Read the model definition and answer for the solid it produces. Units are mm, in the model's axes. Face numbers are marked on the shaded views. Give positions to 0.01 mm unless a question says otherwise; leave off trailing zeros. Order: outer loops, then holes, each group sorted by start corner. A loop starts at its lowest first (then second) coordinate and runs counter-clockwise, first axis right, second up. Notation, with made-up numbers: M 19.25,-17 L 44.25,-17 A20 ccw 44.25,21 Z; hole C 42,21 d7. An arc over 180 degrees is marked long. Write item = value, one per line. Start each with the question number.
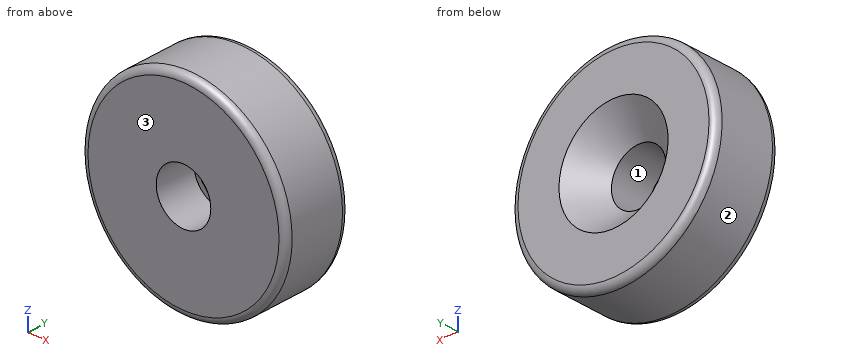
from build123d import *

# Parameters (mm, degrees)
SKETCH1_R           = 7.5
SKETCH1_R_2         = 2
BOSS_EXTRUDE1_DEPTH = 2.5
FILLET1_R           = 0.5
CHAMFER1_SIZE       = 2


with BuildPart() as part:
    # Sketch1 → Boss-Extrude1 (new body, symmetric)
    with BuildSketch(Plane(origin=(0, 0, 0), x_dir=(1, 0, 0), z_dir=(0, 1, 0))):
        Circle(SKETCH1_R)
        Circle(SKETCH1_R_2, mode=Mode.SUBTRACT)
    extrude(amount=BOSS_EXTRUDE1_DEPTH, both=True)

    # Fillet1
    fillet1_edges = [part.edges().sort_by_distance(p)[0] for p in [
        (-7.5, -2.5, 0),
        (-7.5, 2.5, 0),
    ]]
    fillet(fillet1_edges, radius=FILLET1_R)

    # Chamfer1
    chamfer1_edges = [part.edges().sort_by_distance(p)[0] for p in [
        (-2, 2.5, 0),
    ]]
    chamfer(chamfer1_edges, length=CHAMFER1_SIZE)


solid = part.part
1) Find section B-B on x = 0. Determine the outline of the cut face in (y, z), plus the area to 3 significant figures.
2) For a pull along Z with two mould halves and no side action, classify the marked faces 1, 2 and 3 as pulls with the +Z half, pulls with the -Z half, needs draft (parallel to the pull), parting line crosses it, or undercut.
3) Find the intervals of material crossed by probe 1 along X at (y, z) = (-1.05, 0); probe 2 along X at (y, z) = (1.35, 0.25), in increasing order. Write a range as [from, to].
4) Find section C-C on y = -0.45. Determine the outline of the cut face in (x, z), plus the area to 3 significant figures.
5) Find section D-D on y = 1.75. Determine the outline of the cut face in (x, z), plus the area to 3 significant figures.
6) Each of these flat-tipped pins is pushed along its axis until it touches: P1, Ø3, axis at y = -1, z = -6, coming from the +X side; P2, Ø2, axis at x = -4.5, y = 1.5, coming from the +Z side. Where does it stop, or does it pass through?
7) Find section A-A on z = 0. Determine the outline of the cut face in (x, y), plus the area to 3 significant figures.
Numbers:
q1.outline = M -2.5,-7 A0.5 ccw -2,-7.5 L 2,-7.5 A0.5 ccw 2.5,-7 L 2.5,-4 L 0.5,-2 L -2.5,-2 Z; M -2.5,2 L 0.5,2 L 2.5,4 L 2.5,7 A0.5 ccw 2,7.5 L -2,7.5 A0.5 ccw -2.5,7 Z
q1.area = 50.8 mm2
q2.face_1 = undercut
q2.face_2 = parting line crosses it
q2.face_3 = needs draft
q3.probe_1 = [-7.5, -2], [2, 7.5]
q3.probe_2 = [-7.5, -2.84], [2.84, 7.5]
q4.outline = C 0,0 d15; hole C 0,0 d4
q4.area = 164 mm2
q5.outline = C 0,0 d15; hole C 0,0 d6.5
q5.area = 144 mm2
q6.P1 = 6
q6.P2 = 6.63
q7.outline = M -7.5,-2 A0.5 ccw -7,-2.5 L -2,-2.5 L -2,0.5 L -4,2.5 L -7,2.5 A0.5 ccw -7.5,2 Z; M 2,-2.5 L 7,-2.5 A0.5 ccw 7.5,-2 L 7.5,2 A0.5 ccw 7,2.5 L 4,2.5 L 2,0.5 Z
q7.area = 50.8 mm2
